Input: dimensioned drawing with shaded views. Units: mm. Origin: part minimum x, y, z. Give positions to 0.01 mm unless a question says otherwise; leave off trailing zeros. Loops run counter-clockwise (first coordinate to the right, second up) from the corner with the lowest first, then second, coordinate; pieces in that order, holes last. Notation, with made-up numbers: M 82,-31 L 127,-31 A16 cw 127,-23 Z; hole C 80.25,-2.5 d8. An arc over 180 degrees is marked long. Use CSV: the item, a comma, the result in double quotes. Start each with the question number.
Q1. Material intervals for line 1 along X through (y, z) = (1.5, 90); line 2 along X through (y, z) = (1.4, 50); line 3 along Z through (x, y) = (190, 1.3), sorted ascending.
Q2. Section B-B, the plane z = 90. Output: boundary loops of the cut face in (x, y) (3 decimals).
Q3. Section A-A, the plane x = 178. Output: boundary loops of the cut face in (y, z) (3 decimals), plus the area to 3 significant figures.
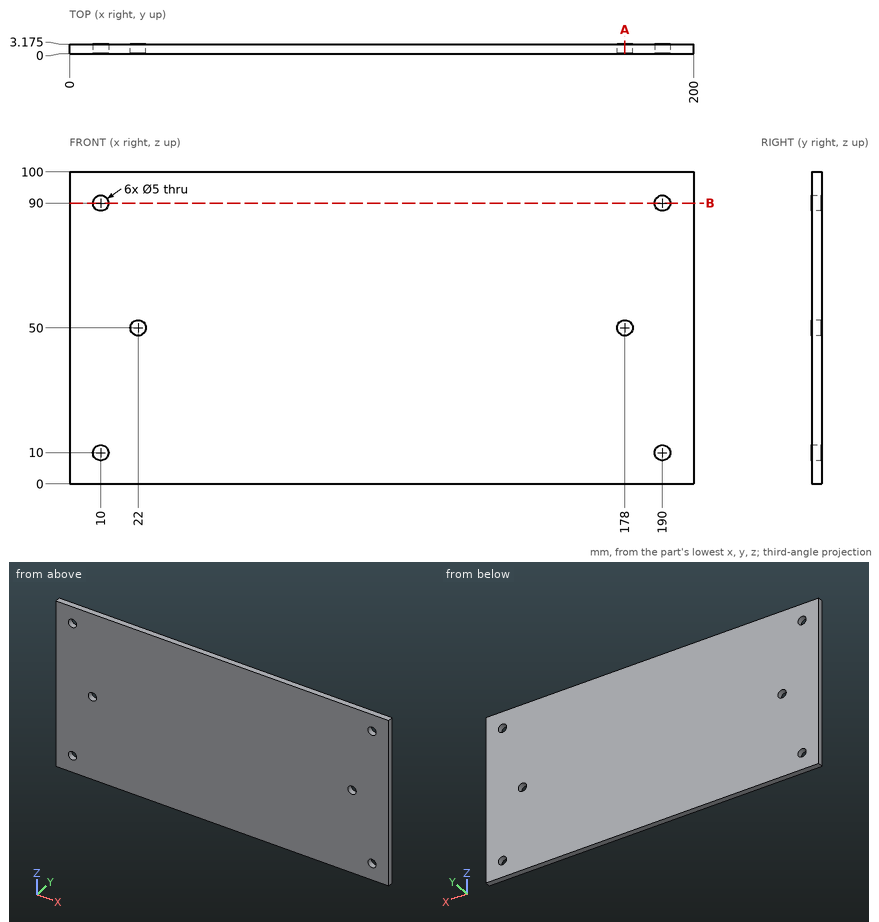
A:
1,line 1,"0 to 7.5, 12.5 to 187.5, 192.5 to 200"
1,line 2,"0 to 19.5, 24.5 to 175.5, 180.5 to 200"
1,line 3,"0 to 7.5, 12.5 to 87.5, 92.5 to 100"
2,outline,"M 0,0 L 7.5,0 L 7.5,3.175 L 0,3.175 Z; M 12.5,0 L 187.5,0 L 187.5,3.175 L 12.5,3.175 Z; M 192.5,0 L 200,0 L 200,3.175 L 192.5,3.175 Z"
3,outline,"M 0,0 L 3.175,0 L 3.175,47.5 L 0,47.5 Z; M 0,52.5 L 3.175,52.5 L 3.175,100 L 0,100 Z"
3,area,"302 mm^2"
